Can you work these out from the model? Positions are in its coordinate system, mm. Face numbers are marked on the shaded views. A direction names the side the tool comes from. Give positions to 0.01 mm unless a question says otherwise; leave off trailing zeros. Write each loop counter-clockwise with the first axis right and the second up, starting at its lowest first coordinate (ties: lowest second). Pieces come first, ordered by that corner, then holes.
```python
from build123d import *

# Parameters (mm, degrees)
SKETCH001_W      = 36.6
SKETCH001_H      = 14.35
EXTRUDE001_DEPTH = 27.6
SKETCH002_W      = 12.7
SKETCH002_H      = 7
POCKET_DEPTH     = 14.351
PAD_DEPTH        = 0.5
SKETCH_W         = 0.6
SKETCH_H         = 0.7
EXTRUDE_DEPTH    = 4.5


with BuildPart() as pad:
    # Sketch001 → Extrude001 (new body)
    with BuildSketch(Plane.XY):
        with Locations((13.97, -0.625)):
            Rectangle(SKETCH001_W, SKETCH001_H)
    extrude(amount=-EXTRUDE001_DEPTH)

    # Sketch002 → Pocket (cut, through all)
    with BuildSketch(Plane(origin=(0, 6.55, 0), x_dir=(-1, 0, 0), z_dir=(0, 1, 0))):
        with Locations((-13.97, -11.8)):
            Rectangle(SKETCH002_W, SKETCH002_H)
    extrude(amount=-POCKET_DEPTH, mode=Mode.SUBTRACT)

    # Sketch003 → Pad (new body)
    with BuildSketch(Plane(origin=(0, 0, -27.6), x_dir=(1, 0, 0), z_dir=(0, 0, -1))):
        Polygon((11.900003, 6.871569), (15.047757, 6.871569), (15.047757, 1.54931), (18.396286, 1.54931), (13.47388, -5.396754), (8.551474, 1.54931), (11.900003, 1.54931), align=None)
    extrude(amount=PAD_DEPTH)


with BuildPart() as fusion:
    # Sketch → Extrude (new body)
    with BuildSketch(Plane.XY):
        Rectangle(SKETCH_W, SKETCH_H)
        with Locations((5.08, 0)):
            Rectangle(SKETCH_W, SKETCH_H)
        with Locations((27.94, 0)):
            Rectangle(SKETCH_W, SKETCH_H)
    extrude(amount=EXTRUDE_DEPTH)

    # Fusion: union Pad
    add(pad.part)


solid = fusion.part
```
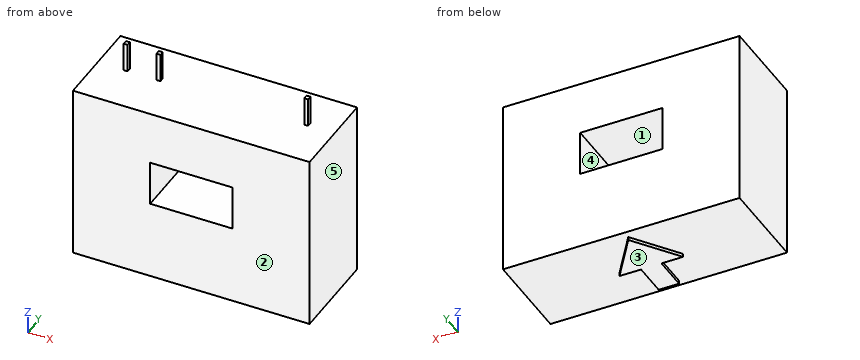
1) Suppose I cut it at C-C on x = 14. Write out the boundary of the cut face in (y, z), plus the area to 3 significant figures.
Values follow:
outline: (-7.8, -27.6) - (-6.87, -27.6) - (-6.87, -28.1) - (4.65, -28.1) - (4.65, -27.6) - (6.55, -27.6) - (6.55, -15.3) - (-7.8, -15.3) - close; (-7.8, -8.3) - (6.55, -8.3) - (6.55, 0) - (-7.8, 0) - close
area: 301 mm2
2) Suppose I cut it at A-A on z = -9. Write out the boundary of the cut face in (x, y).
Values follow:
outline: (-4.33, -7.8) - (7.62, -7.8) - (7.62, 6.55) - (-4.33, 6.55) - close; (20.32, -7.8) - (32.27, -7.8) - (32.27, 6.55) - (20.32, 6.55) - close
3) Suppose I cut it at B-B on y = -3.25. Write out the boundary of the cut face in (x, z).
Values follow:
outline: (-4.33, -27.6) - (11.9, -27.6) - (11.9, -28.1) - (15.05, -28.1) - (15.05, -27.6) - (32.27, -27.6) - (32.27, 0) - (-4.33, 0) - close; hole (7.62, -15.3) - (20.32, -15.3) - (20.32, -8.3) - (7.62, -8.3) - close
4) For pin 1 Ø0.6 at (y, z) = (0, 1) entering from +X; pin 2 Ø0.5 at (x, z) = (28, 3) entering from -Y; pin 3 Ø2 at (x, y) = (25, 1) entering from -Z, each with a flat end and sliding along its axis, tell me the tip position at first contact or that it passes through.
Values follow:
pin 1: stops at x = 28.24
pin 2: stops at y = -0.35
pin 3: stops at z = -27.6
5) For the marked faces 1 and 2, which set-ups out of +Z, -Z, +X, -X, +Y, -Y let a thin tool reach every point of the face, with its end or its side?
Values follow:
face 1: +Y, -Y
face 2: +Z, -Z, +X, -X, -Y
6) Please list where these lines run through material, in increasing order: L1, parallel to Z at x = 18, y = -2.5; L2, parallel to X at y = -3.5, z = -15; L3, parallel to Z at x = 13, y = 4.5.
Values follow:
L1: z = -27.6 to -15.3, -8.3 to 0
L2: x = -4.33 to 7.62, 20.32 to 32.27
L3: z = -28.1 to -15.3, -8.3 to 0
7) Suppose I cut it at D-D on y = 4.5. Write out the boundary of the cut face in (x, z), plus the area to 3 significant figures.
Values follow:
outline: (-4.33, -27.6) - (12.84, -27.6) - (12.84, -28.1) - (14.11, -28.1) - (14.11, -27.6) - (32.27, -27.6) - (32.27, 0) - (-4.33, 0) - close; hole (7.62, -15.3) - (20.32, -15.3) - (20.32, -8.3) - (7.62, -8.3) - close
area: 922 mm2
8) If we mould it in two halves opening along X, with no side actions, what happens to the marked faces 3, 4 and 5? For each: +X half, -X half, draft (parallel to the pull), parting line (faces both ways), or undercut.
Values follow:
face 3: draft
face 4: undercut
face 5: +X half
